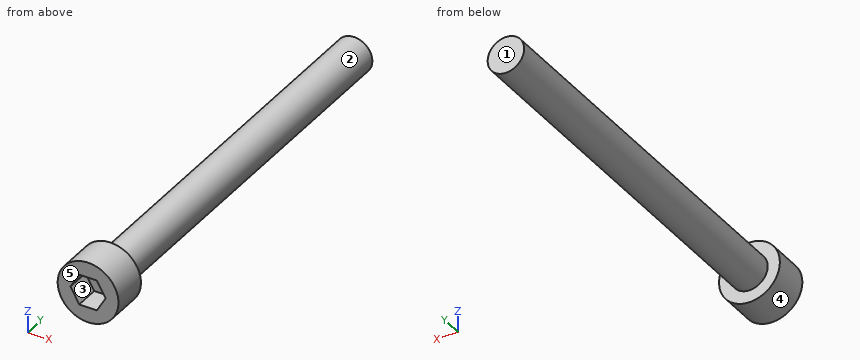
Autodesk Inventor part; units mm, degrees
ref_plane "YZ Plane" through (0, 0, 0) normal (1, 0, 0) x (0, 1, 0)
ref_plane "XZ Plane" through (0, 0, 0) normal (0, 1, 0) x (-1, 0, 0)
ref_plane "XY Plane" through (0, 0, 0) normal (0, 0, 1) x (1, 0, 0)
sketch "Szkic1" plane through (0, 0, 0) normal (0, 1, 0) x (-1, 0, 0)
  circle A0 centre (0, 0) radius 5
  line L0 (1.4434, 2.5) -> (2.8868, 0)
  line L1 (2.8868, 0) -> (1.4434, -2.5)
  line L2 (1.4434, -2.5) -> (-1.4434, -2.5)
  line L3 (-1.4434, -2.5) -> (-2.8868, 0)
  line L4 (-2.8868, 0) -> (-1.4434, 2.5)
  line L5 (-1.4434, 2.5) -> (1.4434, 2.5)
  circle A1 centre (0, 0) radius 3
  dimension "d0" = 10
  dimension "d1" = 5
  dimension "d2" = 6
extrude "Wyciągnięcie proste1" add sketch "Szkic1" along normal blind 2 contours A0 | L0 L1 L2 L3 L4 L5 | A1
extrude "Wyciągnięcie proste2" add sketch "Szkic1" against normal blind 4 contours A0 | A1
sketch "Szkic2" plane through (0, 2, 0) normal (0, 1, 0) x (1, 0, 0)
  circle A0 centre (0, 0) radius 3
  dimension "d7" = 6
extrude "Wyciągnięcie proste3" add sketch "Szkic2" along normal blind 65
thread "Gwint1"
properties part number "M6x65"
Verification items for the finished model (mm, model axes). Face numbers are marked on the shaded views. A direction names the side the tool comes from. Coordinates: 2 decimals unless noted, no trailing zeros. Order: outer loops, then holes, each group sorted by start corner. A loop starts at its lowest first (then second) coordinate and runs counter-clockwise, first axis right, second up. Notation, with made-up numbers: M 57,21 L 72,21 A16 cw 72,38 Z; hole C 21,54 d6. An arc over 180 degrees is marked long. One line per item, written item: value. Start each with the question number.
Item 1: Mould release check, pull along Z, two halves, no side actions. Record for the marked faces 3, 4 and 5: pulls with the +Z half, pulls with the -Z half, needs draft (parallel to the pull), parting line crosses it, or undercut.
Item 2: Sectioned sample at A-A on x = 0. Record the cut outline in (y, z).
Item 3: Sectioned sample at D-D on x = -4. Record the cut outline in (y, z), then the cut area to 3 significant figures.
Item 4: Access from +Z, -Z, +X, -X, +Y, -Y to the whole of each face (thin tool, end or side, straight path). Record for the marked faces 1 and 2.
Item 5: Sectioned sample at C-C on y = 18.5. Record the cut outline in (x, z), then the cut area to 3 significant figures.
Item 6: Sectioned sample at B-B on z = -1.25. Record the cut outline in (x, y), then the cut area to 3 significant figures.
Item 7: Thickness scan on probe 1 along Y at (x, z) = (-4.25, 0.75); probe 2 along Z at (x, y) = (0, 55); probe 3 along Y at (x, z) = (1.75, 0). Record the ranges inside material, lowest first.
Item 8: Depth check by flat-ended pin: P1, Ø5, axis at y = 12, z = -2.5, coming from the -X side; P2, Ø6, axis at x = 4, y = 28, coming from the -Z side; P3, Ø2, axis at x = -2, y = 45.5, coming from the +Z side. Enter the tip coordinate at first touch or a pass-through.
Calculated:
1. face 3: undercut
1. face 4: parting line crosses it
1. face 5: needs draft
2. outline: M -4,-5 L 2,-5 L 2,-3 L 67,-3 L 67,3 L 2,3 L 2,5 L -4,5 L -4,2.5 L 0,2.5 L 0,-2.5 L -4,-2.5 Z
3. outline: M -4,-3 L 2,-3 L 2,3 L -4,3 Z
3. area: 36.0 mm^2
4. face 1: +Z, -Z, +X, -X, +Y
4. face 2: +Y
5. outline: C 0,0 d6
5. area: 28.3 mm^2
6. outline: M -4.84,-4 L -2.17,-4 L -2.17,0 L 2.17,0 L 2.17,-4 L 4.84,-4 L 4.84,2 L 2.73,2 L 2.73,67 L -2.73,67 L -2.73,2 L -4.84,2 Z
6. area: 395 mm^2
7. probe 1: -4 to 2
7. probe 2: -3 to 3
7. probe 3: 0 to 67
8. P1: x = -3
8. P2: z = -2.83
8. P3: z = 2.83
